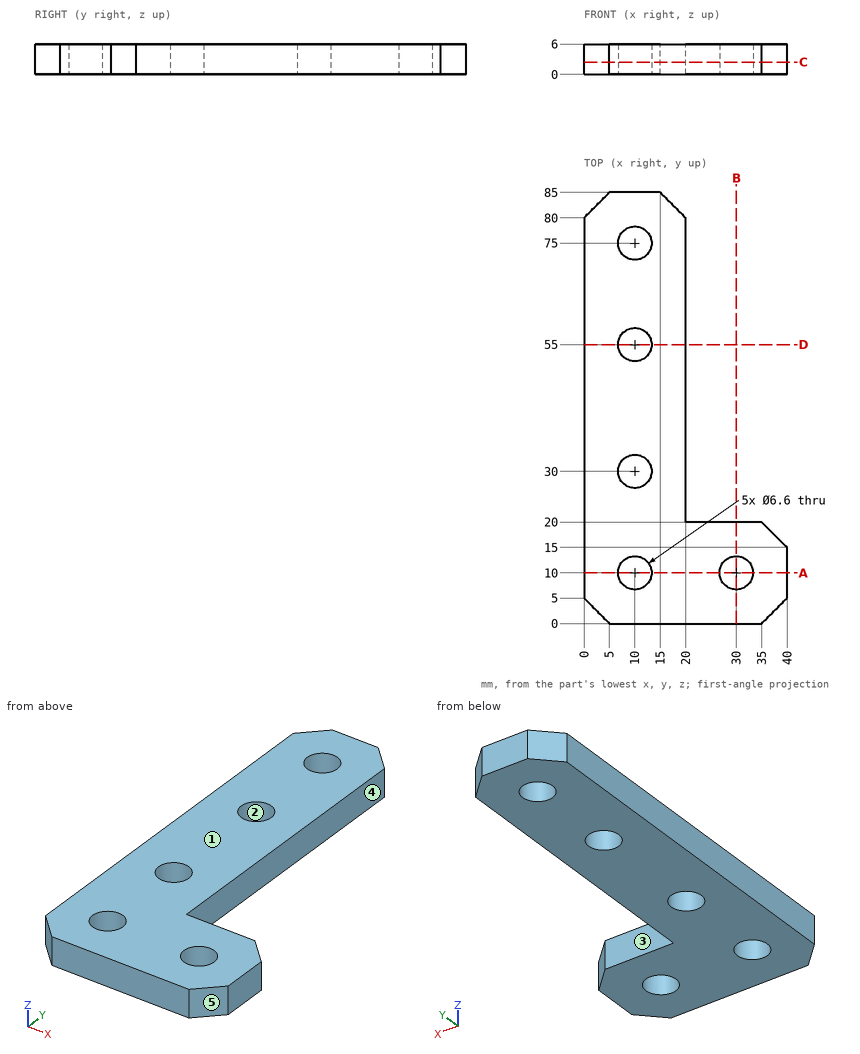
Study the drawing (mm; zero at the part's minimum x, y, z) and answer. A direction names the side the tool comes from. Round coordinates to 2 decimals unless told otherwise and drop trailing zeros. Loops run counter-clockwise (first coordinate to the right, second up) from the corner with the lowest first, then second, coordinate; pieces in that order, holes last. Notation, with made-up numbers: (60, 26) - (85, 26) arc R8 ccw to (85, 31) - close; hole circle Ø2 at (-5.75, 14.5). An arc over 180 degrees is marked (long way). Use one line per item in the form item = value. Start each with the question number.
1. Given pin 1 Ø1 at (y, z) = (46.5, 4.5) entering from +X; pin 2 Ø1.5 at (x, z) = (32, 2.5) entering from +Y, each flat-ended and moving along its own axis, determine where each tip first touches the part or whether it passes through.
2. The part is cut by section C-C on z = 2.45. Determine the outline of the cut face in (x, y), then the cut area to 3 significant figures.
3. A tool of negligible diameter and unlimited length cuts with its end or side. For the marked faces 4 and 5, from which of +Z, -Z, +X, -X, +Y, -Y can it reach the whole face along a straight path? Write none if from no direction.
4. Consider line 1 (Y direction, x = 10, z = 1.3); line 2 (X direction, y = 11.5, z = 5.3); line 3 (X direction, y = 9, z = 3). Determine where each line is inside the solid, lowest interval first. Write a range as [from, to].
5. For a pull along Y with two mould halves and no side action, classify the marked faces 1, 2 and 3 as pulls with the +Y half, pulls with the -Y half, needs draft (parallel to the pull), parting line crosses it, or undercut.
6. The part is cut by section A-A on y = 10. Determine the outline of the cut face in (x, z), then the cut area to 3 significant figures.
7. The part is cut by section B-B on x = 30. Determine the outline of the cut face in (y, z), then the cut area to 3 significant figures.
Geometry check:
q1.pin_1 = 20
q1.pin_2 = 20
q2.outline = (0, 5) - (5, 0) - (35, 0) - (40, 5) - (40, 15) - (35, 20) - (20, 20) - (20, 80) - (15, 85) - (5, 85) - (0, 80) - close; hole circle Ø6.6 at (10, 10); hole circle Ø6.6 at (10, 30); hole circle Ø6.6 at (10, 55); hole circle Ø6.6 at (10, 75); hole circle Ø6.6 at (30, 10)
q2.area = 1,870 mm^2
q3.face_4 = +Z, -Z, +X, +Y
q3.face_5 = +Z, -Z, +X, -Y
q4.line_1 = [0, 6.7], [13.3, 26.7], [33.3, 51.7], [58.3, 71.7], [78.3, 85]
q4.line_2 = [0, 7.06], [12.94, 27.06], [32.94, 40]
q4.line_3 = [0, 6.86], [13.14, 26.86], [33.14, 40]
q5.face_1 = needs draft
q5.face_2 = undercut
q5.face_3 = pulls with the +Y half
q6.outline = (0, 0) - (6.7, 0) - (6.7, 6) - (0, 6) - close; (13.3, 0) - (26.7, 0) - (26.7, 6) - (13.3, 6) - close; (33.3, 0) - (40, 0) - (40, 6) - (33.3, 6) - close
q6.area = 161 mm^2
q7.outline = (0, 0) - (6.7, 0) - (6.7, 6) - (0, 6) - close; (13.3, 0) - (20, 0) - (20, 6) - (13.3, 6) - close
q7.area = 80.4 mm^2
